Could you check a few things on this model? Use its own coordinates, in mm. A direction names the side the tool comes from. Round coordinates to 2 decimals unless told otherwise and drop trailing zeros. Loops run counter-clockwise (first coordinate to the right, second up) from the corner with the lowest first, then second, coordinate; pieces in that order, holes last. Notation, with made-up numbers: (-33.5, 52.25) -> (21.5, 52.25) arc R18 cw to (21.5, 70.25) -> close; hole circle Ø4 at (83, 64). An arc over 180 degrees is marked (long way). Write each question's results on one line, items separated by ' | '.
from build123d import *

# Parameters (mm, degrees)
SKETCH1_W           = 20
SKETCH1_H           = 8
BOSS_EXTRUDE1_DEPTH = 115
CUT_EXTRUDE1_DEPTH  = 60
SKETCH3_W           = 20
SKETCH3_H           = 115
BOSS_EXTRUDE2_DEPTH = 3
SKETCH13_W          = 46.736094472
SKETCH13_H          = 63.842099498
CUT_EXTRUDE5_DEPTH  = 30
SKETCH15_W          = 20
SKETCH15_H          = 40
CUT_EXTRUDE6_DEPTH  = 6
FILLET1_R           = 5


with BuildPart() as part:
    # Sketch1 → Boss-Extrude1 (new body)
    with BuildSketch(Plane.XY):
        with Locations((-16.536312849, 6.223463687)):
            Rectangle(SKETCH1_W, SKETCH1_H)
    extrude(amount=-BOSS_EXTRUDE1_DEPTH)

    # Sketch2 → Cut-Extrude1 (cut)
    with BuildSketch(Plane.XY):
        Polygon((-26.536312849, 7.723463687), (-22.186312849, 7.723463687), (-22.186312849, 5.723463687), (-23.686312849, 5.723463687), (-23.686312849, 4.223463687), (-22.186312849, 4.223463687), (-22.186312849, 2.723463687), (-20.536312849, 2.723463687), (-20.536312849, 7.723463687), (-12.536312849, 7.723463687), (-12.536312849, 2.723463687), (-10.886312849, 2.723463687), (-10.886312849, 4.223463687), (-9.386312849, 4.223463687), (-9.386312849, 5.723463687), (-10.886312849, 5.723463687), (-10.886312849, 7.723463687), (-6.536312849, 7.723463687), (-6.536312849, 2.223463687), (-26.536312849, 2.223463687), align=None)
    extrude(amount=-CUT_EXTRUDE1_DEPTH, mode=Mode.SUBTRACT)

    # Sketch3 → Boss-Extrude2 (add)
    with BuildSketch(Plane(origin=(0, 10.223463687, 0), x_dir=(1, 0, 0), z_dir=(0, 1, 0))):
        with Locations((-16.536312849, 57.5)):
            Rectangle(SKETCH3_W, SKETCH3_H)
    extrude(amount=BOSS_EXTRUDE2_DEPTH)

    # Sketch13 → Cut-Extrude5 (cut)
    with BuildSketch(Plane(origin=(0, -39.878862952, -23.02407226), x_dir=(-1, 0, 0), z_dir=(0, 0.866025403784438, 0.500000000000001))):
        with Locations((16.217588554, -100.321082734)):
            Rectangle(SKETCH13_W, SKETCH13_H)
    extrude(amount=-CUT_EXTRUDE5_DEPTH, mode=Mode.SUBTRACT)

    # Sketch15 → Cut-Extrude6 (cut)
    with BuildSketch(Plane.XZ.offset(-2.223463687)):
        with Locations((-16.536312849, -87)):
            Rectangle(SKETCH15_W, SKETCH15_H)
    extrude(amount=-CUT_EXTRUDE6_DEPTH, mode=Mode.SUBTRACT)

    # Fillet1
    fillet1_edges = [part.edges().sort_by_distance(p)[0] for p in [
        (-16.536312849, 2.223463687, -67),
    ]]
    fillet(fillet1_edges, radius=FILLET1_R)


solid = part.part
1) I want a section at D-D, the plane z = -91. Write out the boundary of the cut face in (x, y), plus the area to 3 significant figures.
Model answer:
outline: (-26.54, 8.22) -> (-6.54, 8.22) -> (-6.54, 13.22) -> (-26.54, 13.22) -> close | area: 100 mm2
2) I need wall thicknesses on line 1 (X direction, y = 7.5, z = -55); line 2 (Y direction, x = -13.75, z = -55); line 3 (X direction, y = 5.25, z = -44). Which ranges of each line are inside material? Lowest first, please.
Model answer:
line 1: x = -22.19 to -20.54, -12.54 to -10.89 | line 2: y = 7.72 to 13.22 | line 3: x = -23.69 to -20.54, -12.54 to -9.39
3) I'm going to push flat-ended pins straight in: pin 1 (1.6 mm diameter, centred on y = 5, z = -27.5, fed in from +X); pin 2 (5 mm diameter, centred on x = -10, y = 7.5, fed in from -Z); pin 3 (0.8 mm diameter, centred on x = -23, z = -34, fed in from -Y). Where does each tip first touch, or does it pass through?
Model answer:
pin 1: stops at x = -9.39 | pin 2: stops at z = -109.42 | pin 3: stops at y = 4.22
4) For faces 4 (the flat face through (-17, 8.223, -86)), 5 (the flat face through (-24, 7.723, -30)), 6 (the flat face through (-9, 7.723, -30)), 7 (the flat face through (-17, 7.723, -30)), which set-ups out of +Z, -Z, +X, -X, +Y, -Y let a thin tool reach every point of the face, with its end or its side?
Model answer:
face 4: -Z, +X, -X, -Y | face 5: +Z, -X | face 6: +Z, +X | face 7: +Z, -Y
5) If we mould it in two halves opening along X, with no side actions, what happens to faces 1 (the flat face through (-20.536, 5, -30)), 2 (the flat face through (-16.4, 10.69, -110.61)), 3 (the flat face through (-26.536, 11, -57))? For each: released by +X, released by -X, zero draft, split by the parting line, or undercut.
Model answer:
face 1: undercut | face 2: zero draft | face 3: released by -X
6) I want a section at C-C, the plane y = 11. Write out the boundary of the cut face in (x, z).
Model answer:
outline: (-26.54, -111.15) -> (-6.54, -111.15) -> (-6.54, 0) -> (-26.54, 0) -> close
7) I want a section at A-A, the plane x = -14.75. Write out the boundary of the cut face in (y, z).
Model answer:
outline: (2.22, -62) arc R5 ccw to (7.22, -67) -> (8.22, -67) -> (8.22, -106.34) -> (13.22, -115) -> (13.22, 0) -> (7.72, 0) -> (7.72, -60) -> (2.22, -60) -> close
8) I want a section at B-B, the plane z = -33.5. Write out the boundary of the cut face in (x, y), plus the area to 3 significant figures.
Model answer:
outline: (-26.54, 7.72) -> (-22.19, 7.72) -> (-22.19, 5.72) -> (-23.69, 5.72) -> (-23.69, 4.22) -> (-22.19, 4.22) -> (-22.19, 2.72) -> (-20.54, 2.72) -> (-20.54, 7.72) -> (-12.54, 7.72) -> (-12.54, 2.72) -> (-10.89, 2.72) -> (-10.89, 4.22) -> (-9.39, 4.22) -> (-9.39, 5.72) -> (-10.89, 5.72) -> (-10.89, 7.72) -> (-6.54, 7.72) -> (-6.54, 13.22) -> (-26.54, 13.22) -> close | area: 131 mm2
